```python
from build123d import *

# Parameters (mm, degrees)
MODEL_R             = 2.6
MODEL_R_2           = 1.1
BOSS_EXTRUDE1_DEPTH = 7


with BuildPart() as part:
    # Model → Boss-Extrude1 (new body)
    with BuildSketch(Plane.XY):
        with BuildLine():
            Line((3, 0), (41, 0))
            ThreePointArc((41, 0), (43.121320344, -0.878679656), (44, -3))
            Line((44, -3), (44, -42))
            ThreePointArc((44, -42), (43.121320344, -44.121320344), (41, -45))
            Line((41, -45), (23, -45))
            ThreePointArc((23, -45), (20.878679656, -45.878679656), (20, -48))
            Line((20, -48), (20, -66))
            ThreePointArc((20, -66), (19.121320344, -68.121320344), (17, -69))
            Line((17, -69), (3, -69))
            ThreePointArc((3, -69), (0.878679656, -68.121320344), (0, -66))
            Line((0, -66), (0, -3))
            ThreePointArc((0, -3), (0.878679656, -0.878679656), (3, 0))
        make_face()
        with Locations((34, -8)):
            Circle(MODEL_R, mode=Mode.SUBTRACT)
        with Locations((34, -37)):
            Circle(MODEL_R, mode=Mode.SUBTRACT)
        with Locations((5.4, -59)):
            Circle(MODEL_R_2, mode=Mode.SUBTRACT)
        with Locations((15, -59)):
            Circle(MODEL_R_2, mode=Mode.SUBTRACT)
    extrude(amount=BOSS_EXTRUDE1_DEPTH)


solid = part.part
```
Build history of the part. All positions in model axes, mm. A direction names the side the tool comes from. Give positions to 0.01 mm unless a question says otherwise; leave off trailing zeros. Loops run counter-clockwise (first coordinate to the right, second up) from the corner with the lowest first, then second, coordinate; pieces in that order, holes last. Notation, with made-up numbers: (72, -1) - (120, -1) arc R18 ccw to (120, 4) - close; hole circle Ø9 at (-4.5, 62). An arc over 180 degrees is marked (long way). Use a Markdown table: item, result.
(1) Wall check: line 1 along Y through (x, z) = (34, 5.5); line 2 along Y through (x, z) = (15, 2.25); line 3 along X through (y, z) = (-57, 1.25). Give the ranges that are in metal, low to high.
Taken from the geometry:
| item | result |
|---|---|
| line 1 | -45 to -39.6, -34.4 to -10.6, -5.4 to 0 |
| line 2 | -69 to -60.1, -57.9 to 0 |
| line 3 | 0 to 20 |
(2) Which spindle directions (+Z, -Z, +X, -X, +Y, -Y) get a long thin tool onto all of the face, cutting with end or side? Do faces 1 (the face through (31.937, -38.582, 3.451)), 2 (the face through (20, -57, 3)). Say none if no direction does.
Taken from the geometry:
| item | result |
|---|---|
| face 1 | +Z, -Z |
| face 2 | +Z, -Z, +X, -Y |
(3) Band-saw the part on B-B (x = 15). Give the cut face in (y, z).
Taken from the geometry:
| item | result |
|---|---|
| outline | (-69, 0) - (-60.1, 0) - (-60.1, 7) - (-69, 7) - close; (-57.9, 0) - (0, 0) - (0, 7) - (-57.9, 7) - close |
(4) Band-saw the part on D-D (z = 6). Give the cut face in (x, y).
Taken from the geometry:
| item | result |
|---|---|
| outline | (0, -66) arc R3 ccw to (3, -69) - (17, -69) arc R3 ccw to (20, -66) - (20, -48) arc R3 cw to (23, -45) - (41, -45) arc R3 ccw to (44, -42) - (44, -3) arc R3 ccw to (41, 0) - (3, 0) arc R3 ccw to (0, -3) - close; hole circle Ø2.2 at (5.4, -59); hole circle Ø2.2 at (15, -59); hole circle Ø5.2 at (34, -37); hole circle Ø5.2 at (34, -8) |
(5) Band-saw the part on A-A (x = 34). Give the cut face in (y, z), and give its area (3 significant figures).
Taken from the geometry:
| item | result |
|---|---|
| outline | (-45, 0) - (-39.6, 0) - (-39.6, 7) - (-45, 7) - close; (-34.4, 0) - (-10.6, 0) - (-10.6, 7) - (-34.4, 7) - close; (-5.4, 0) - (0, 0) - (0, 7) - (-5.4, 7) - close |
| area | 242 mm2 |
(6) Band-saw the part on C-C (y = -37). Give the cut face in (x, z).
Taken from the geometry:
| item | result |
|---|---|
| outline | (0, 0) - (31.4, 0) - (31.4, 7) - (0, 7) - close; (36.6, 0) - (44, 0) - (44, 7) - (36.6, 7) - close |
(7) Drop flat-ended pins along their axis: pin 1 Ø3.5 at (y, z) = (-60.5, 2) entering from +X; pin 2 Ø2 at (x, z) = (32.5, 3.5) entering from -Y. Give the stop position or say it passes through.
Taken from the geometry:
| item | result |
|---|---|
| pin 1 | x = 20 |
| pin 2 | y = -45 |
(8) Pull direction X, two halves, no side cores. Call faces 3 (the face through (5.99, -58.07, 3.45)), 4 (the face through (22, 0, 3)), 5 (the face through (0.9, -68.14, 3.45)): +X half, -X half, draft (parallel to the pull), parting line (faces both ways), or undercut.
Taken from the geometry:
| item | result |
|---|---|
| face 3 | undercut |
| face 4 | draft |
| face 5 | -X half |
